```python
from build123d import *

# Parameters (mm, degrees)
BOX_W               = 70
BOX_H               = 200
BOX_DEPTH           = 11.6
POCKET_DEPTH        = 200.001
LINEARPATTERN_COUNT = 6
LINEARPATTERN_PITCH = 10
SKETCH_W            = 82.408782
SKETCH_H            = 38.885188
SKETCH_W_2          = 45.5
SKETCH_H_2          = 14.501198
POCKET001_DEPTH     = 200.001
SKETCH003_R         = 1
POCKET002_DEPTH     = 11.601
CHAMFER_SIZE        = 1
FILLET_R            = 0.92


with BuildPart() as part:
    # Box → Box (new body)
    with BuildSketch(Plane(origin=(-7.5, 0, 0), x_dir=(1, 0, 0), z_dir=(0, 0, 1))):
        with Locations((35, 100)):
            Rectangle(BOX_W, BOX_H)
    extrude(amount=BOX_DEPTH)

    # Sketch002 → Pocket (cut, through all)
    with BuildSketch(Plane(origin=(-7.5, 0, 0), x_dir=(1, 0, 0), z_dir=(0, -1, 0))):
        Polygon((10.05, 10), (7.25, 10), (7.25, 3), (2.75, 3), (2.75, 10), (1.95, 10), (1.95, 10.4), (2.25, 11.6), (9.75, 11.6), (10.05, 10.4), align=None)
    pocket = extrude(amount=-POCKET_DEPTH, mode=Mode.SUBTRACT)

    # LinearPattern: Pocket ×6
    with Locations(*[(i * LINEARPATTERN_PITCH, 0, 0) for i in range(1, LINEARPATTERN_COUNT)]):
        add(pocket, mode=Mode.SUBTRACT)

    # Sketch → Pocket001 (cut, through all)
    with BuildSketch(Plane(origin=(-7.5, 0, 0), x_dir=(1, 0, 0), z_dir=(0, -1, 0))):
        with Locations((35.413628, 6.289411)):
            Rectangle(SKETCH_W, SKETCH_H)
        with Locations((30, 5.862397)):
            Rectangle(SKETCH_W_2, SKETCH_H_2, mode=Mode.SUBTRACT)
    extrude(amount=-POCKET001_DEPTH, mode=Mode.SUBTRACT)

    # Sketch003 → Pocket002 (cut, through all)
    with BuildSketch(Plane(origin=(-7.5, 0, 0), x_dir=(1, 0, 0), z_dir=(0, 0, -1))):
        with Locations((15, -10)):
            Circle(SKETCH003_R)
        with Locations((45, -10)):
            Circle(SKETCH003_R)
        with Locations((15, -190)):
            Circle(SKETCH003_R)
        with Locations((45, -190)):
            Circle(SKETCH003_R)
        with Locations((15, -100)):
            Circle(SKETCH003_R)
        with Locations((45, -100)):
            Circle(SKETCH003_R)
    extrude(amount=-POCKET002_DEPTH, mode=Mode.SUBTRACT)

    # Chamfer
    chamfer_edges = [part.edges().sort_by_distance(p)[0] for p in [
        (36.5, 190, 3),
        (6.5, 190, 3),
        (36.5, 100, 3),
        (6.5, 100, 3),
        (36.5, 10, 3),
        (6.5, 10, 3),
    ]]
    chamfer(chamfer_edges, length=CHAMFER_SIZE)

    # Fillet
    fillet_edges = [part.edges().sort_by_distance(p)[0] for p in [
        (1.15, 0, 10),
        (2.55, 0, 10.2),
        (2.4, 0, 11),
        (4.6, 0, 11),
        (4.45, 0, 10.2),
        (4.85, 0, 10),
        (11.15, 0, 10),
        (12.55, 0, 10.2),
        (12.4, 0, 11),
        (14.6, 0, 11),
        (14.45, 0, 10.2),
        (14.85, 0, 10),
        (21.15, 0, 10),
        (22.55, 0, 10.2),
        (22.4, 0, 11),
        (24.6, 0, 11),
        (24.45, 0, 10.2),
        (24.85, 0, 10),
        (31.15, 0, 10),
        (32.55, 0, 10.2),
        (32.4, 0, 11),
        (34.6, 0, 11),
        (34.45, 0, 10.2),
        (34.85, 0, 10),
        (41.15, 0, 10),
        (42.55, 0, 10.2),
        (42.4, 0, 11),
        (44.6, 0, 11),
        (44.45, 0, 10.2),
        (44.85, 0, 10),
        (1.15, 200, 10),
        (2.55, 200, 10.2),
        (2.4, 200, 11),
        (4.85, 200, 10),
        (4.45, 200, 10.2),
        (4.6, 200, 11),
        (11.15, 200, 10),
        (12.55, 200, 10.2),
        (12.4, 200, 11),
        (14.6, 200, 11),
        (14.45, 200, 10.2),
        (14.85, 200, 10),
        (21.15, 200, 10),
        (22.55, 200, 10.2),
        (22.4, 200, 11),
        (24.6, 200, 11),
        (24.45, 200, 10.2),
        (24.85, 200, 10),
        (31.15, 200, 10),
        (32.55, 200, 10.2),
        (32.4, 200, 11),
        (34.6, 200, 11),
        (34.45, 200, 10.2),
        (34.85, 200, 10),
        (41.15, 200, 10),
        (42.55, 200, 10.2),
        (42.4, 200, 11),
        (44.6, 200, 11),
        (44.45, 200, 10.2),
        (44.85, 200, 10),
    ]]
    fillet(fillet_edges, radius=FILLET_R)


solid = part.part
```
Check sheet for the modelled part. Datum: model origin and axes. Units: mm. A direction names the side the tool comes from. Coordinates: 2 decimals unless noted, no trailing zeros.
1) Access from +Z, -Z, +X, -X, +Y, -Y to the whole of each face (thin tool, end or side, straight path). Record for faces 1 (the face through (29.75, 99, 7)), 2 (the face through (22, 0, 4)).
2) Material ranges on probe 1 along Y at (x, z) = (37.5, 0.6); probe 2 along X at (y, z) = (161, 9), recorded low to high.
3) Gauge pin test, flat end, axial feed: pin 1 (3.5 mm diameter, centred on x = 38.5, y = 98.5, fed in from +Z). Record the tip position at first contact, or that the pin passes through.
Check sheet entries:
1. face 1: +Z, +Y, -Y
1. face 2: +Z, -Z, +X, -X, -Y
2. probe 1: y = 0 to 9, 11 to 99, 101 to 189, 191 to 200
2. probe 2: x = -0.25 to 5.25, 9.75 to 15.25, 19.75 to 25.25, 29.75 to 35.25, 39.75 to 45.25
3. pin 1: stops at z = 10
